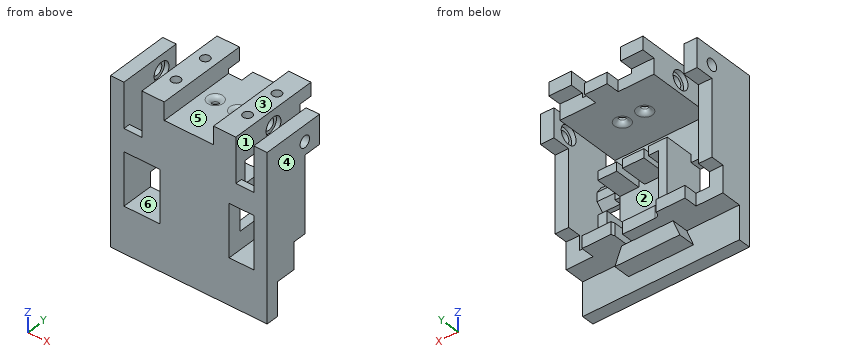
from build123d import *

# Parameters (mm, degrees)
BOSS_EXTRUDE1_DEPTH  = 20.5
SKETCH5_W            = 23
SKETCH5_H            = 23
BOSS_EXTRUDE3_DEPTH  = 6
BOSS_EXTRUDE6_DEPTH  = 18
SKETCH18_W           = 2.6
SKETCH18_H           = 4
SKETCH18_W_2         = 2
SKETCH18_W_3         = 4
SKETCH18_H_2         = 15
SKETCH18_H_3         = 5.5
CUT_EXTRUDE10_DEPTH  = 14.5
SKETCH8_W            = 6
SKETCH8_H            = 13
BOSS_EXTRUDE4_DEPTH  = 8
SKETCH7_R            = 2.575
CUT_EXTRUDE_X_DEPTH  = 6
SKETCH9_R            = 4.05
CUT_EXTRUDE4_DEPTH   = 2
SKETCH10_W           = 29
SKETCH10_H           = 13
BOSS_EXTRUDE5_DEPTH  = 28.5
SKETCH12_W           = 8
SKETCH12_H           = 13
CUT_EXTRUDE6_DEPTH   = 24
SKETCH13_R           = 2.575
CUT_EXTRUDE7_DEPTH   = 6
SKETCH14_R           = 4.05
CUT_EXTRUDE8_DEPTH   = 2
CUT_EXTRUDE21_REACH  = 61
SKETCH35_R           = 1.5
CUT_EXTRUDE22_REACH  = 30.5
FILLET1_R            = 2
BOSS_EXTRUDE7_DEPTH  = 12.5
SKETCH34_R           = 2.05
CUT_EXTRUDE20_DEPTH  = 10
SKETCH38_W           = 70
SKETCH38_H           = 5.5
BOSS_EXTRUDE8_DEPTH  = 15
BOSS_EXTRUDE9_DEPTH  = 7.5
CUT_EXTRUDE23_START  = -5.5
CUT_EXTRUDE23_DEPTH  = 5.5
BOSS_EXTRUDE10_DEPTH = 58
CUT_EXTRUDE24_REACH  = 76
SKETCH42_W           = 8
SKETCH42_H           = 4.5
BOSS_EXTRUDE11_START = -14
SKETCH43_W           = 10
SKETCH43_H           = 5
BOSS_EXTRUDE11_DEPTH = 42
BOSS_EXTRUDE12_REACH = 22
SKETCH44_W           = 42
SKETCH44_H           = 5
SKETCH45_W           = 12
SKETCH45_H           = 12
CUT_EXTRUDE25_DEPTH  = 6
CUT_EXTRUDE26_DEPTH  = 6


with BuildPart() as part:
    # Sketch1 → Boss-Extrude1 (new body)
    with BuildSketch(Plane(origin=(0, 0, 0), x_dir=(1, 0, 0), z_dir=(0, 1, 0))):
        Polygon((-29, 24), (-29, -29.5), (-35, -29.5), (-35, 29.5), (35, 29.5), (35, -29.5), (29, -29.5), (29, 24), align=None)
    extrude(amount=-BOSS_EXTRUDE1_DEPTH)



with BuildPart() as body_2:
    # Sketch5 → Boss-Extrude3 (new body)
    with BuildSketch(Plane(origin=(0, -20.5, 0), x_dir=(1, 0, 0), z_dir=(0, 1, 0))):
        with Locations((2.5, 12.5)):
            Rectangle(SKETCH5_W, SKETCH5_H)
    extrude(amount=BOSS_EXTRUDE3_DEPTH)


with BuildPart() as part_1:
    add(part.part)

    add(body_2.part)  # Boss-Extrude6 merges body 2
    # Sketch16 → Boss-Extrude6 (add)
    with BuildSketch(Plane.XZ.offset(20.5)):
        Polygon((18, -24), (14, -24), (14, -1), (-9, -1), (-9, -24), (-13, -24), (-13, 3), (18, 3), align=None)
    extrude(amount=-BOSS_EXTRUDE6_DEPTH)

    # Sketch18 → Cut-Extrude10 (cut)
    with BuildSketch(Plane(origin=(0, 0, 0), x_dir=(1, 0, 0), z_dir=(0, 1, 0))):
        with Locations((8.25, -1)):
            Rectangle(SKETCH18_W, SKETCH18_H)
        with Locations((-3.55, -1)):
            Rectangle(SKETCH18_W_2, SKETCH18_H)
        with Locations((16, 8.5)):
            Rectangle(SKETCH18_W_3, SKETCH18_H_2)
        with Locations((8.25, 26.75)):
            Rectangle(SKETCH18_W, SKETCH18_H_3)
    extrude(amount=-CUT_EXTRUDE10_DEPTH, mode=Mode.SUBTRACT)

    # Sketch8 → Boss-Extrude4 (add)
    with BuildSketch(Plane(origin=(0, 0, 0), x_dir=(1, 0, 0), z_dir=(0, 1, 0))):
        with Locations((32, -23)):
            Rectangle(SKETCH8_W, SKETCH8_H)
    boss_extrude4 = extrude(amount=BOSS_EXTRUDE4_DEPTH)

    # Sketch7 → Cut-Extrude x (cut)
    with BuildSketch(Plane(origin=(35, 0, 0), x_dir=(0, 0, -1), z_dir=(1, 0, 0))):
        with Locations((-22.291637032, 0)):
            Circle(SKETCH7_R)
    cut_extrude_x = extrude(amount=-CUT_EXTRUDE_X_DEPTH, mode=Mode.SUBTRACT)

    # Sketch9 → Cut-Extrude4 (cut)
    with BuildSketch(Plane(origin=(29, 0, 0), x_dir=(0, 0, -1), z_dir=(1, 0, 0))):
        with Locations((-22.291637032, 0)):
            Circle(SKETCH9_R)
    cut_extrude4 = extrude(amount=CUT_EXTRUDE4_DEPTH, mode=Mode.SUBTRACT)

    # Sketch10 → Boss-Extrude5 (add)
    with BuildSketch(Plane.XZ.offset(20.5)):
        with Locations((14.5, 23)):
            Rectangle(SKETCH10_W, SKETCH10_H)
    boss_extrude5 = extrude(amount=-BOSS_EXTRUDE5_DEPTH)

    # Sketch12 → Cut-Extrude6 (cut)
    with BuildSketch(Plane(origin=(0, 8, 0), x_dir=(1, 0, 0), z_dir=(0, 1, 0))):
        with Locations((25, -23)):
            Rectangle(SKETCH12_W, SKETCH12_H)
    cut_extrude6 = extrude(amount=-CUT_EXTRUDE6_DEPTH, mode=Mode.SUBTRACT)

    # Sketch13 → Cut-Extrude7 (cut)
    with BuildSketch(Plane(origin=(21, 0, 0), x_dir=(0, 0, -1), z_dir=(1, 0, 0))):
        with Locations((-22.291637032, 0)):
            Circle(SKETCH13_R)
    cut_extrude7 = extrude(amount=-CUT_EXTRUDE7_DEPTH, mode=Mode.SUBTRACT)

    # Sketch14 → Cut-Extrude8 (cut)
    with BuildSketch(Plane(origin=(21, 0, 0), x_dir=(0, 0, -1), z_dir=(1, 0, 0))):
        with Locations((-22.291637032, 0)):
            Circle(SKETCH14_R)
    cut_extrude8 = extrude(amount=-CUT_EXTRUDE8_DEPTH, mode=Mode.SUBTRACT)

    # Mirror1: Boss-Extrude4, Cut-Extrude x, Cut-Extrude4, Boss-Extrude5, Cut-Extrude6, Cut-Extrude7, Cut-Extrude8 across plane
    add(boss_extrude4.mirror(Plane(origin=(0, 0, 0), x_dir=(0, 0, 1), z_dir=(1, 0, 0))))
    add(cut_extrude_x.mirror(Plane(origin=(0, 0, 0), x_dir=(0, 0, 1), z_dir=(1, 0, 0))), mode=Mode.SUBTRACT)
    add(cut_extrude4.mirror(Plane(origin=(0, 0, 0), x_dir=(0, 0, 1), z_dir=(1, 0, 0))), mode=Mode.SUBTRACT)
    add(boss_extrude5.mirror(Plane(origin=(0, 0, 0), x_dir=(0, 0, 1), z_dir=(1, 0, 0))))
    add(cut_extrude6.mirror(Plane(origin=(0, 0, 0), x_dir=(0, 0, 1), z_dir=(1, 0, 0))), mode=Mode.SUBTRACT)
    add(cut_extrude7.mirror(Plane(origin=(0, 0, 0), x_dir=(0, 0, 1), z_dir=(1, 0, 0))), mode=Mode.SUBTRACT)
    add(cut_extrude8.mirror(Plane(origin=(0, 0, 0), x_dir=(0, 0, 1), z_dir=(1, 0, 0))), mode=Mode.SUBTRACT)

    # Sketch35 → Cut-Extrude21 (cut, up to next)
    with BuildSketch(Plane.XY.offset(29.5), mode=Mode.PRIVATE) as cut_extrude21_sk1:
        with Locations((-5, 0)):
            Circle(SKETCH35_R)
    cut_extrude21_tool1 = extrude(cut_extrude21_sk1.sketch, amount=-CUT_EXTRUDE21_REACH, mode=Mode.PRIVATE) & part_1.part
    add(cut_extrude21_tool1.solids().sort_by_distance((-5, 0, 29.5))[0], mode=Mode.SUBTRACT)
    # Sketch35 → Cut-Extrude21 (cut, up to next)
    with BuildSketch(Plane.XY.offset(29.5), mode=Mode.PRIVATE) as cut_extrude21_sk2:
        with Locations((5, 0)):
            Circle(SKETCH35_R)
    cut_extrude21_tool2 = extrude(cut_extrude21_sk2.sketch, amount=-CUT_EXTRUDE21_REACH, mode=Mode.PRIVATE) & part_1.part
    add(cut_extrude21_tool2.solids().sort_by_distance((5, 0, 29.5))[0], mode=Mode.SUBTRACT)

    # Sketch36 → Cut-Extrude22 (cut, up to next)
    with BuildSketch(Plane(origin=(0, 8, 0), x_dir=(1, 0, 0), z_dir=(0, 1, 0)), mode=Mode.PRIVATE) as cut_extrude22_sk1:
        Polygon((-5, -29.5), (5, -29.5), (11, -29.5), (11, -21.5), (-11, -21.5), (-11, -29.5), align=None)
    cut_extrude22_tool1 = extrude(cut_extrude22_sk1.sketch, amount=-CUT_EXTRUDE22_REACH, mode=Mode.PRIVATE) & part_1.part
    add(cut_extrude22_tool1.solids().sort_by_distance((0, 8, 25.5))[0], mode=Mode.SUBTRACT)

    # Fillet1
    fillet1_edges = [part_1.edges().sort_by_distance(p)[0] for p in [
        (-6.5, 0, 16.5),
        (3.5, 0, 16.5),
        (-6.5, 0, 21.5),
        (3.5, 0, 21.5),
    ]]
    fillet(fillet1_edges, radius=FILLET1_R)

    # Sketch37 → Boss-Extrude7 (add)
    with BuildSketch(Plane(origin=(0, 8, 0), x_dir=(1, 0, 0), z_dir=(0, 1, 0))):
        Polygon((-11, -21.5), (11, -21.5), (11, -29.5), (21, -29.5), (21, -16.5), (-21, -16.5), (-21, -29.5), (-11, -29.5), align=None)
    extrude(amount=BOSS_EXTRUDE7_DEPTH)

    # Sketch34 → Cut-Extrude20 (cut)
    with BuildSketch(Plane.XY.offset(29.5)):
        with Locations((16, -8)):
            Circle(SKETCH34_R)
        with Locations((16, 8)):
            Circle(SKETCH34_R)
        with Locations((-16, 8)):
            Circle(SKETCH34_R)
        with Locations((-16, -8)):
            Circle(SKETCH34_R)
    extrude(amount=-CUT_EXTRUDE20_DEPTH, mode=Mode.SUBTRACT)

    # Sketch38 → Boss-Extrude8 (add)
    with BuildSketch(Plane(origin=(0, 0, -29.5), x_dir=(-1, 0, 0), z_dir=(0, 0, -1))):
        with Locations((0, -17.75)):
            Rectangle(SKETCH38_W, SKETCH38_H)
    extrude(amount=BOSS_EXTRUDE8_DEPTH)

    # Sketch39 → Boss-Extrude9 (add)
    with BuildSketch(Plane(origin=(0, -15, 0), x_dir=(1, 0, 0), z_dir=(0, 1, 0))):
        Polygon((11.5, 29.5), (14.5, 37), (-14.5, 37), (-11.5, 29.5), align=None)
    extrude(amount=BOSS_EXTRUDE9_DEPTH)

    # Sketch40 → Cut-Extrude23 (cut)
    with BuildSketch(Plane(origin=(0, 0, -29.5), x_dir=(-1, 0, 0), z_dir=(0, 0, -1)).offset(CUT_EXTRUDE23_START)):
        with BuildLine():
            Line((-7.5, 2.5), (7.5, 2.5))
            ThreePointArc((7.5, 2.5), (10, 0), (7.5, -2.5))
            Line((7.5, -2.5), (-7.5, -2.5))
            ThreePointArc((-7.5, -2.5), (-10, 0), (-7.5, 2.5))
        make_face()
    extrude(amount=CUT_EXTRUDE23_DEPTH, mode=Mode.SUBTRACT)

    # Sketch41 → Boss-Extrude10 (add)
    with BuildSketch(Plane.ZY.offset(-29)):
        Polygon((-0.5, -20.5), (9.5, -20.5), (9.5, -17.5), (6.5, -15.5), (2.5, -15.5), (-0.5, -18.5), align=None)
    extrude(amount=BOSS_EXTRUDE10_DEPTH)

    # Sketch42 → Cut-Extrude24 (cut, up to next)
    with BuildSketch(Plane.XY.offset(29.5), mode=Mode.PRIVATE) as cut_extrude24_sk1:
        with Locations((25, -18.25)):
            Rectangle(SKETCH42_W, SKETCH42_H)
    cut_extrude24_tool1 = extrude(cut_extrude24_sk1.sketch, amount=-CUT_EXTRUDE24_REACH, mode=Mode.PRIVATE) & part_1.part
    add(cut_extrude24_tool1.solids().sort_by_distance((25, -18.25, 29.5))[0], mode=Mode.SUBTRACT)
    # Sketch42 → Cut-Extrude24 (cut, up to next)
    with BuildSketch(Plane.XY.offset(29.5), mode=Mode.PRIVATE) as cut_extrude24_sk2:
        with Locations((-25, -18.25)):
            Rectangle(SKETCH42_W, SKETCH42_H)
    cut_extrude24_tool2 = extrude(cut_extrude24_sk2.sketch, amount=-CUT_EXTRUDE24_REACH, mode=Mode.PRIVATE) & part_1.part
    add(cut_extrude24_tool2.solids().sort_by_distance((-25, -18.25, 29.5))[0], mode=Mode.SUBTRACT)

    # Sketch43 → Boss-Extrude11 (add)
    with BuildSketch(Plane(origin=(35, 0, 0), x_dir=(0, 0, -1), z_dir=(1, 0, 0)).offset(BOSS_EXTRUDE11_START)):
        with Locations((-4.5, -18)):
            Rectangle(SKETCH43_W, SKETCH43_H)
    extrude(amount=-BOSS_EXTRUDE11_DEPTH)

    # Sketch44 → Boss-Extrude12 (add, up to next)
    with BuildSketch(Plane.XY.offset(9.5), mode=Mode.PRIVATE) as boss_extrude12_sk1:
        with Locations((0, -18)):
            Rectangle(SKETCH44_W, SKETCH44_H)
    boss_extrude12_tool1 = extrude(boss_extrude12_sk1.sketch, amount=BOSS_EXTRUDE12_REACH, mode=Mode.PRIVATE) - part_1.part
    add(boss_extrude12_tool1.solids().sort_by_distance((0, -18, 9.5))[0])

    # Sketch45 → Cut-Extrude25 (cut)
    with BuildSketch(Plane(origin=(0, 0, 0), x_dir=(1, 0, 0), z_dir=(0, 1, 0))):
        with Locations((29, 23.5)):
            Rectangle(SKETCH45_W, SKETCH45_H)
        with Locations((-29, 23.5)):
            Rectangle(SKETCH45_W, SKETCH45_H)
    extrude(amount=-CUT_EXTRUDE25_DEPTH, mode=Mode.SUBTRACT)

    # Sketch46 → Cut-Extrude26 (cut)
    with BuildSketch(Plane(origin=(0, 20.5, 0), x_dir=(1, 0, 0), z_dir=(0, 1, 0))):
        Polygon((-5, -21.5), (-5, -16.5), (-21, -16.5), (-21, -23.5), (-11, -23.5), (-11, -21.5), align=None)
        Polygon((5, -21.5), (5, -16.5), (21, -16.5), (21, -23.5), (11, -23.5), (11, -21.5), align=None)
    extrude(amount=-CUT_EXTRUDE26_DEPTH, mode=Mode.SUBTRACT)


solid = part_1.part
Input: part model. Units: mm. Frame: model coordinates. Face numbers are marked on the shaded views. A direction names the side the tool comes from. Coordinates: 2 decimals unless noted, no trailing zeros. Loops run counter-clockwise (first coordinate to the right, second up) from the corner with the lowest first, then second, coordinate; pieces in that order, holes last.
Q1. Cut plane C-C (y = 16). Output: boundary loops of the cut face in (x, z).
Q2. Contact query for flat-ended pins moving along their axis: pin 1 (2 mm diameter, centred on x = 6, y = -12.5, fed in from -Z); pin 2 (4 mm diameter, centred on x = 0.5, z = -32.5, fed in from +Y); pin 3 (1.2 mm diameter, centred on x = 15, z = 0, fed in from +Y); pin 4 (1 mm diameter, centred on x = -22.5, y = 11, fed in from +Z). Output: stop coordinate, or through.
Q3. Cut plane B-B (x = -16). Output: boundary loops of the cut face in (y, z) (3 decimals).
Q4. Material intervals for line 1 (Z direction, x = -6, y = -12); line 2 (Y direction, x = -16, z = 25); line 3 (X direction, y = -11.5, z = -6), sorted ascending.
Q5. Cut plane D-D (x = -30). Output: boundary loops of the cut face in (y, z).
Q6. Draft query along Z for the marked faces 1, 2 and 3. Return one class per face: +Z half, -Z half, draft (parallel to the pull), parting line (faces both ways), or undercut.
Q7. Cut plane A-A (z = 14). Output: boundary loops of the cut face in (x, y), then the cut area to 3 significant figures.
Q8. Set-up query: the marked faces 4, 5 and 6. Return all of +Z, -Z, +X, -X, +Y, -Y with unobstructed straight access to the full face (end or side cutting, diameter ignored); none if empty.
Working result:
1. outline: (-21, 23.5) - (-11, 23.5) - (-11, 29.5) - (-21, 29.5) - close; (-5, 16.5) - (5, 16.5) - (5, 21.5) - (-5, 21.5) - close; (11, 23.5) - (21, 23.5) - (21, 29.5) - (11, 29.5) - close
2. pin 1: stops at z = -37
2. pin 2: stops at y = -7.5
2. pin 3: stops at y = -2.5
2. pin 4: passes through
3. outline: (-20.5, -44.5) - (-15, -44.5) - (-15, -29.5) - (0, -29.5) - (0, -24) - (-20.5, -24) - close; (-20.5, -0.5) - (-15.5, -0.5) - (-15.5, 16.5) - (14.5, 16.5) - (14.5, 23.5) - (20.5, 23.5) - (20.5, 29.5) - (10.05, 29.5) - (10.05, 19.5) - (5.95, 19.5) - (5.95, 29.5) - (-5.95, 29.5) - (-5.95, 19.5) - (-10.05, 19.5) - (-10.05, 29.5) - (-20.5, 29.5) - close; hole circle Ø5.15 at (0, 22.292)
4. line 1: z = -37 to -24, -1 to 3, 16.5 to 21.5
4. line 2: y = -20.5 to -10.05, -5.95 to 5.95, 10.05 to 20.5
4. line 3: x = -35 to -29, -13 to -9, 29 to 35
5. outline: (-20.5, -44.5) - (-15, -44.5) - (-15, -29.5) - (-6, -29.5) - (-6, -17.5) - (0, -17.5) - (0, 16.5) - (8, 16.5) - (8, 29.5) - (-20.5, 29.5) - close; hole circle Ø8.1 at (0, 22.29)
6. face 1: draft
6. face 2: undercut
6. face 3: +Z half
7. outline: (-35, -20.5) - (-29, -20.5) - (-29, 0) - (-35, 0) - close; (-21, -20.5) - (21, -20.5) - (21, -15.5) - (-21, -15.5) - close; (29, -20.5) - (35, -20.5) - (35, 0) - (29, 0) - close
7. area: 456 mm2
8. face 4: +Z, -Z, +X, +Y, -Y
8. face 5: +Z, +Y, -Y
8. face 6: +Y
